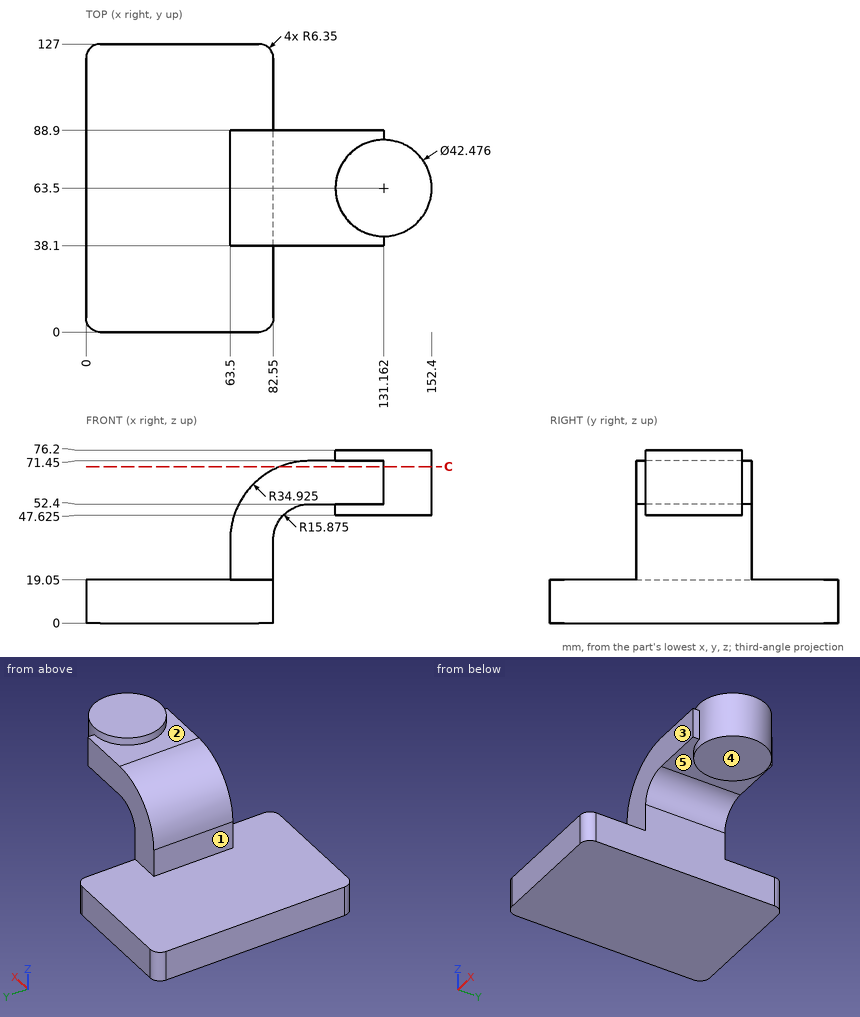
Answer from the drawing. Dimensions are ordinates in mm from the lowest x, y and z of the part. A direction names the side the tool comes from. Coordinates: 2 decimals unless noted, no trailing zeros. Order: outer loops, then holes, each group sorted by start corner. A loop starts at its lowest first (then second) coordinate and runs counter-clockwise, first axis right, second up. Notation, with made-up numbers: (46.25, 10) - (86.25, 10) arc R17 ccw to (86.25, 29) - close; hole circle Ø3 at (2.5, 4.25). An arc over 180 degrees is marked (long way). Put each result on its own line as item: value. Start each with the question number.
1) For the marked faces 1, 2, 3, 4 and 5, determine the directions among +Z, -Z, +X, -X, +Y, -Y from which every point of the face is accessible in a straight line to the end or side of a thin tool.
2) Find the intervals of material crossed by line 1 (Z direction, x = 48, y = 32); line 2 (Z direction, x = 143, y = 71) (1 decimal); line 3 (Y direction, x = 70, z = 32), in increasing order. Write a range as from..to.
3) Flat-ended cylindrical pins translate along their axes: pin 1 (10 mm diameter, centred on y = 69.5, z = 24, fed in from +X); pin 2 (6 mm diameter, centred on x = 78, y = 88, fed in from +Z); pin 3 (5 mm diameter, centred on y = 53.5, z = 24, fed in from -X). Find the tip coordinate at first contact, or state that the pin passes through.
4) Find section C-C (z = 69). Give the vertices of the cut face in (x, y) (1 decimal), plus the area to 3 significant figures.
Results list:
1. face 1: +Z, -X, +Y, -Y
1. face 2: +Z, -X
1. face 3: +Z, +X, -X, -Y
1. face 4: -Z, +X, +Y, -Y
1. face 5: -Z
2. line 1: z = 0..19.05
2. line 2: z = 47.6..76.2
2. line 3: y = 38.1..88.9
3. pin 1: stops at x = 82.55
3. pin 2: stops at z = 66.79
3. pin 3: stops at x = 63.5
4. outline: (85.6, 38.1) - (131.2, 38.1) - (131.2, 42.3) arc R21.2 ccw to (131.2, 84.7) - (131.2, 88.9) - (85.6, 88.9) - close
4. area: 3,020 mm^2
